from build123d import *

# Parameters (mm, degrees)
F0_W     = 25
F0_H     = 20
F0_H_2   = 5
F0_W_2   = 20
F0_H_3   = 25
F1_DEPTH = 25
F2_W     = 20
F2_H     = 20
F3_DEPTH = 20
F4_W     = 20
F4_H     = 20
F5_DEPTH = 20
F6_W     = 25
F6_H     = 25
F6_W_2   = 20
F6_H_2   = 20
F7_DEPTH = 20


with BuildPart() as f1:
    # F0 (on Top) → F1 (new body)
    with BuildSketch(Plane.XY):
        with Locations((-12.5, 20)):
            Rectangle(F0_W, F0_H)
        Polygon((5, 30), (0, 30), (0, 10), (0, 5), (5, 5), align=None)
        with Locations((-12.5, 7.5)):
            Rectangle(F0_W, F0_H_2)
        with Locations((15, 17.5)):
            Rectangle(F0_W_2, F0_H_3)
    extrude(amount=F1_DEPTH)

    # F2 (on face) → F3 (cut)
    with BuildSketch(Plane(origin=(0, 30, 0), x_dir=(-1, 0, 0), z_dir=(0, 1, 0))):
        with Locations((12.5, 12.5)):
            Rectangle(F2_W, F2_H)
    extrude(amount=-F3_DEPTH, mode=Mode.SUBTRACT)

    # F4 (on face) → F5 (cut)
    with BuildSketch(Plane.YZ.offset(25)):
        with Locations((17.5, 12.5)):
            Rectangle(F4_W, F4_H)
    extrude(amount=-F5_DEPTH, mode=Mode.SUBTRACT)

    # F6 (on face) → F7 (join)
    with BuildSketch(Plane.XY.offset(25)):
        with Locations((-12.5, 17.5)):
            Rectangle(F6_W, F6_H)
        with Locations((-12.5, 17.5)):
            Rectangle(F6_W_2, F6_H_2, mode=Mode.SUBTRACT)
    extrude(amount=F7_DEPTH)


solid = f1.part
Work out the finished part from the listing and answer in its coordinate system (mm). A direction names the side the tool comes from. Give positions to 0.01 mm unless a question says otherwise; leave off trailing zeros. Order: outer loops, then holes, each group sorted by start corner. A loop starts at its lowest first (then second) coordinate and runs counter-clockwise, first axis right, second up. Notation, with made-up numbers: (27, -27) - (71, -27) arc R32 ccw to (71, 1) - close; hole circle Ø1 at (64, 34.5). An arc over 180 degrees is marked (long way). Answer as CSV lines item,"result". Start each with the question number.
Q1. The part is cut by section B-B (x = 14). Write down the section's boundary in (y, z), then the cut area to 3 significant figures.
Q2. The mould has two halves that part along X. Classify faces 5 (the face through (25, 28, 12)), 6 (the face through (-6, 5, 17)), 7 (the face through (-12, 20, 2.5)): +X half, -X half, draft (parallel to the pull), parting line (faces both ways), or undercut.
Q3. For faces 1 (the face through (-13, 27.5, 35)), 2 (the face through (-2.5, 20, 12)), 3 (the face through (15, 17, 22.5)), 4 (the face through (12, 18, 25)), determine the directions among +Z, -Z, +X, -X, +Y, -Y from which every point of the face is accessible in a straight line to the end or side of a thin tool.
Q4. The part is cut by section A-A (y = 12). Write down the section's boundary in (x, z).
Q5. Find the intervals of material crossed by L1, parallel to X at y = 20.75, z = 41.5; L2, parallel to Z at x = 7, y = 14.5; L3, parallel to X at y = 25.75, z = 13, in increasing order. Write a range as [from, to].
Q6. Given pin 1 Ø12 at (x, y) = (-14, 19) entering from +Z; pin 2 Ø1 at (y, z) = (25, 16) entering from +X; pin 3 Ø5 at (x, z) = (-5.5, 17.5) entering from +Y, each flat-ended and moving along its own axis, determine where each tip first touches the part or whether it passes through.
Q7. The part is cut by section C-C (z = 17.5). Write down the section's boundary in (x, y), then the cut area to 3 significant figures.
Q8. The part is cut by section D-D (z = 27.5). Write down the section's boundary in (x, y).
Check result:
1,outline,"(5, 0) - (30, 0) - (30, 25) - (5, 25) - close; hole (7.5, 2.5) - (27.5, 2.5) - (27.5, 22.5) - (7.5, 22.5) - close"
1,area,"225 mm²"
2,face 5,"+X half"
2,face 6,"draft"
2,face 7,"undercut"
3,face 1,"+Z"
3,face 2,"+Y"
3,face 3,"+X"
3,face 4,"+Z, +X, +Y, -Y"
4,outline,"(-25, 0) - (25, 0) - (25, 2.5) - (5, 2.5) - (5, 22.5) - (25, 22.5) - (25, 25) - (0, 25) - (0, 45) - (-2.5, 45) - (-2.5, 25) - (-22.5, 25) - (-22.5, 45) - (-25, 45) - close; hole (-22.5, 2.5) - (-2.5, 2.5) - (-2.5, 22.5) - (-22.5, 22.5) - close"
5,L1,"x = [-25, -22.5], [-2.5, 0]"
5,L2,"z = [0, 2.5], [22.5, 25]"
5,L3,"x = [-25, -22.5], [-2.5, 5]"
6,pin 1,"stops at z = 25"
6,pin 2,"stops at x = 5"
6,pin 3,"stops at y = 10"
7,outline,"(-25, 5) - (25, 5) - (25, 7.5) - (5, 7.5) - (5, 27.5) - (25, 27.5) - (25, 30) - (-2.5, 30) - (-2.5, 10) - (-22.5, 10) - (-22.5, 30) - (-25, 30) - close"
7,area,"450 mm²"
8,outline,"(-25, 5) - (0, 5) - (0, 30) - (-25, 30) - close; hole (-22.5, 7.5) - (-2.5, 7.5) - (-2.5, 27.5) - (-22.5, 27.5) - close"
